from build123d import *

# Parameters (mm, degrees)
F0_W         = 97
F0_H         = 67
F1_DEPTH     = 5
F0_W_2       = 107
F0_H_2       = 77
F2_DEPTH     = 47
F3_R         = 10
F4_T1_DEPTH  = 87
F4_T3_DEPTH  = 57
F4_T6_ANGLE  = 90
F4_T8_ANGLE  = 90
F4_T10_ANGLE = 90
F4_T12_ANGLE = 90


# Not quite as in the source:
# - a fillet or chamfer that OpenCascade refuses, or shapes differently, is made with other operations: its cross-section is extruded or revolved along the edge and cut away or added


with BuildPart() as f1:
    # F0 (on Top) → F1 (new body)
    with BuildSketch(Plane.XY):
        Rectangle(F0_W, F0_H)
    extrude(amount=F1_DEPTH)

    # F0 (on Top) → F2 (join)
    with BuildSketch(Plane.XY):
        Rectangle(F0_W_2, F0_H_2)
        Rectangle(F0_W, F0_H, mode=Mode.SUBTRACT)
    extrude(amount=F2_DEPTH)

    # F3
    f3_edges = [f1.edges().sort_by_distance(p)[0] for p in [
        (-53.5, 38.5, 23.5),
        (53.5, 38.5, 23.5),
        (53.5, -38.5, 23.5),
        (-53.5, -38.5, 23.5),
    ]]
    fillet(f3_edges, radius=F3_R)

    # F4: fillet of radius 5 on 8 edges, made by hand

    # F4_s2 → F4_t1 (cut)
    with BuildSketch(Plane.YZ.offset(-43.5)):
        with BuildLine():
            ThreePointArc((-38.5, 42), (-37.0355339059, 45.5355339059), (-33.5, 47))
            Line((-33.5, 47), (-38.5, 47))
            Line((-38.5, 47), (-38.5, 42))
        make_face()
        with BuildLine():
            ThreePointArc((38.5, 42), (37.0355339059, 45.5355339059), (33.5, 47))
            Line((33.5, 47), (38.5, 47))
            Line((38.5, 47), (38.5, 42))
        make_face()
    extrude(amount=F4_T1_DEPTH, mode=Mode.SUBTRACT)

    # F4_s4 → F4_t3 (cut)
    with BuildSketch(Plane.XZ.offset(-28.5)):
        with BuildLine():
            ThreePointArc((53.5, 42), (52.0355339059, 45.5355339059), (48.5, 47))
            Line((48.5, 47), (53.5, 47))
            Line((53.5, 47), (53.5, 42))
        make_face()
        with BuildLine():
            ThreePointArc((-53.5, 42), (-52.0355339059, 45.5355339059), (-48.5, 47))
            Line((-48.5, 47), (-53.5, 47))
            Line((-53.5, 47), (-53.5, 42))
        make_face()
    extrude(amount=F4_T3_DEPTH, mode=Mode.SUBTRACT)

    # F4_s5 → F4_t6 (revolve, cut)
    with BuildSketch(Plane.YZ.offset(43.5)):
        with BuildLine():
            ThreePointArc((38.5, 42), (37.0355339059, 45.5355339059), (33.5, 47))
            Line((33.5, 47), (38.5, 47))
            Line((38.5, 47), (38.5, 42))
        make_face()
    revolve(axis=Axis((43.5, 28.5, 47), (0, 0, -1)), revolution_arc=F4_T6_ANGLE, mode=Mode.SUBTRACT)

    # F4_s7 → F4_t8 (revolve, cut)
    with BuildSketch(Plane.YZ.offset(-43.5)):
        with BuildLine():
            ThreePointArc((38.5, 42), (37.0355339059, 45.5355339059), (33.5, 47))
            Line((33.5, 47), (38.5, 47))
            Line((38.5, 47), (38.5, 42))
        make_face()
    revolve(axis=Axis((-43.5, 28.5, 47), (0, 0, 1)), revolution_arc=F4_T8_ANGLE, mode=Mode.SUBTRACT)

    # F4_s9 → F4_t10 (revolve, cut)
    with BuildSketch(Plane.YZ.offset(43.5)):
        with BuildLine():
            ThreePointArc((-38.5, 42), (-37.0355339059, 45.5355339059), (-33.5, 47))
            Line((-33.5, 47), (-38.5, 47))
            Line((-38.5, 47), (-38.5, 42))
        make_face()
    revolve(axis=Axis((43.5, -28.5, 47), (0, 0, 1)), revolution_arc=F4_T10_ANGLE, mode=Mode.SUBTRACT)

    # F4_s11 → F4_t12 (revolve, cut)
    with BuildSketch(Plane.XZ.offset(28.5)):
        with BuildLine():
            ThreePointArc((-53.5, 42), (-52.0355339059, 45.5355339059), (-48.5, 47))
            Line((-48.5, 47), (-53.5, 47))
            Line((-53.5, 47), (-53.5, 42))
        make_face()
    revolve(axis=Axis((-43.5, -28.5, 47), (0, 0, 1)), revolution_arc=F4_T12_ANGLE, mode=Mode.SUBTRACT)


solid = f1.part
Here's how the part is built. I have some questions about the finished solid (model axes, mm). A direction names the side the tool comes from. Round coordinates to 2 decimals unless told otherwise and drop trailing zeros. Loops run counter-clockwise (first coordinate to the right, second up) from the corner with the lowest first, then second, coordinate; pieces in that order, holes last.
1. If we section it at B-B on y = 16.5: Write out the boundary of the cut face in (x, z).
Answer list:
outline: (-53.5, 0) - (53.5, 0) - (53.5, 42) arc R5 ccw to (48.5, 47) - (48.5, 5) - (-48.5, 5) - (-48.5, 47) arc R5 ccw to (-53.5, 42) - close
2. For P1, Ø2, axis at x = -7.5, y = 13, coming from the +Z side; P2, Ø1.5, axis at y = -30.5, z = 39.5, coming from the +X side, each with a flat end and sliding along its axis, tell me the tip position at first contact or that it passes through.
Answer list:
P1: stops at z = 5
P2: stops at x = 53.42
3. If we section it at C-C on x = -38.5: Write out the boundary of the cut face in (y, z), plus the area to 3 significant figures.
Answer list:
outline: (-38.5, 0) - (38.5, 0) - (38.5, 42) arc R5 ccw to (33.5, 47) - (33.5, 5) - (-33.5, 5) - (-33.5, 47) arc R5 ccw to (-38.5, 42) - close
area: 794 mm2
4. Which directions (+Z, -Z, +X, -X, +Y, -Y) give clear straight access to the entire face, cutting with the end or side of a thin tool? Please do faces 1 (the face through (-1, -38.5, 21)), 2 (the face through (-1, 0, 5)).
Answer list:
face 1: +Z, -Z, +X, -X, -Y
face 2: +Z
5. If I drill on line 1 along Y through (x, z) = (37, 10.5); line 2 along X through (y, z) = (-4, 19); line 3 along Z through (x, y) = (-22, 19), over which ranges is the centre line in solid material (lowest first)?
Answer list:
line 1: y = -38.5 to -33.5, 33.5 to 38.5
line 2: x = -53.5 to -48.5, 48.5 to 53.5
line 3: z = 0 to 5
6. We'd pull the mould along Y, two halves only. Please class faces 3 (the face through (-1, 38.5, 21)), 4 (the face through (-52.07, 0.4, 45.5)), 5 (the face through (-1, 33.5, 26)): +Y half, -Y half, draft (parallel to the pull), parting line (faces both ways), or undercut.
Answer list:
face 3: +Y half
face 4: draft
face 5: undercut
7. If we section it at A-A on z = 29: Write out the boundary of the cut face in (x, y), plus the area to 3 significant figures.
Answer list:
outline: (-53.5, -28.5) arc R10 ccw to (-43.5, -38.5) - (43.5, -38.5) arc R10 ccw to (53.5, -28.5) - (53.5, 28.5) arc R10 ccw to (43.5, 38.5) - (-43.5, 38.5) arc R10 ccw to (-53.5, 28.5) - close; hole (-48.5, -33.5) - (48.5, -33.5) - (48.5, 33.5) - (-48.5, 33.5) - close
area: 1,650 mm2
